from build123d import *

# Parameters (mm, degrees)
F0_W     = 43.040663
F0_H     = 37.921667
F1_DEPTH = 25.4
F2_R     = 5.08
F3_R     = 3.052253
F4_DEPTH = 25.4


with BuildPart() as f1:
    # F0 (on Top) → F1 (new body)
    with BuildSketch(Plane.XY):
        with Locations((21.520331, 18.960833)):
            Rectangle(F0_W, F0_H)
    extrude(amount=F1_DEPTH)

    # F2
    f2_edges = [f1.edges().sort_by_distance(p)[0] for p in [
        (43.040663, 18.960834, 0),
        (21.520332, 37.921667, 0),
        (21.520332, 0, 0),
        (0, 18.960834, 0),
        (43.040663, 18.960834, 25.4),
        (43.040663, 37.921667, 12.7),
        (43.040663, 0, 12.7),
        (0, 0, 12.7),
        (0, 37.921667, 12.7),
        (21.520332, 37.921667, 25.4),
        (21.520332, 0, 25.4),
        (0, 18.960834, 25.4),
    ]]
    fillet(f2_edges, radius=F2_R)

    # F3 (on face) → F4 (cut)
    with BuildSketch(Plane.XY.offset(25.4)):
        with Locations((22.265185, 18.770991)):
            Circle(F3_R)
    extrude(amount=-F4_DEPTH, mode=Mode.SUBTRACT)


solid = f1.part
For this review, take the finished solid that the model builds, in its own axes (mm). Round coordinates to 2 decimals unless told otherwise and drop trailing zeros. Write each loop counter-clockwise with the first axis right and the second up, starting at its lowest first coordinate (ties: lowest second). Pieces come first, ordered by that corner, then holes. Notation, with made-up numbers: (-21.5, -35) - (-4.5, -35) arc R24 ccw to (-4.5, -17) - close; hole circle Ø4 at (22, 85). An arc over 180 degrees is marked (long way). Write item = value, one per line. Start each with the question number.
1. Consider section A-A on z = 8. State the section outline as (x, y) points.
2. Consider section B-B on x = 9.5. State the section outline as (y, z) points.
3. Draft analysis for pull direction Y (two halves, no side actions). For faces 1 (the face through (25.176, 19.688, 12.878)), 2 (the face through (21, 37.922, 13)), 3 (the face through (41.513, 1.449, 12.807)), 4 (the face through (43.041, 19, 13)), state which applies: released by +Y, released by -Y, zero draft, split by the parting line, or undercut.
4. Wall thickness on L1, parallel to Z at x = 30, y = 5; L2, parallel to X at y = 19.5, z = 14.25; L3, parallel to X at y = 5, z = 14.75: over which ranges is each line inside the solid? List them lowest first.
5. Consider section C-C on y = 9.5. State the section outline as (x, z) points, plus the area to 3 significant figures.
6. For pin 1 Ø2 at (x, z) = (20, 21.5) entering from +Y; pin 2 Ø5 at (x, y) = (22.27, 18.77) entering from -Z, all flat-tipped, find the tip position at first contact; note any pin that passes through.
Evaluation:
q1.outline = (0, 5.08) arc R5.08 ccw to (5.08, 0) - (37.96, 0) arc R5.08 ccw to (43.04, 5.08) - (43.04, 32.84) arc R5.08 ccw to (37.96, 37.92) - (5.08, 37.92) arc R5.08 ccw to (0, 32.84) - close; hole circle Ø6.1 at (22.27, 18.77)
q2.outline = (0, 5.08) arc R5.08 ccw to (5.08, 0) - (32.84, 0) arc R5.08 ccw to (37.92, 5.08) - (37.92, 20.32) arc R5.08 ccw to (32.84, 25.4) - (5.08, 25.4) arc R5.08 ccw to (0, 20.32) - close
q3.face_1 = undercut
q3.face_2 = released by +Y
q3.face_3 = released by -Y
q3.face_4 = zero draft
q4.L1 = 0 to 25.4
q4.L2 = 0 to 19.3, 25.23 to 43.04
q4.L3 = 0 to 43.04
q5.outline = (0, 5.08) arc R5.08 ccw to (5.08, 0) - (37.96, 0) arc R5.08 ccw to (43.04, 5.08) - (43.04, 20.32) arc R5.08 ccw to (37.96, 25.4) - (5.08, 25.4) arc R5.08 ccw to (0, 20.32) - close
q5.area = 1,070 mm2
q6.pin_1 = 37.92
q6.pin_2 = through
